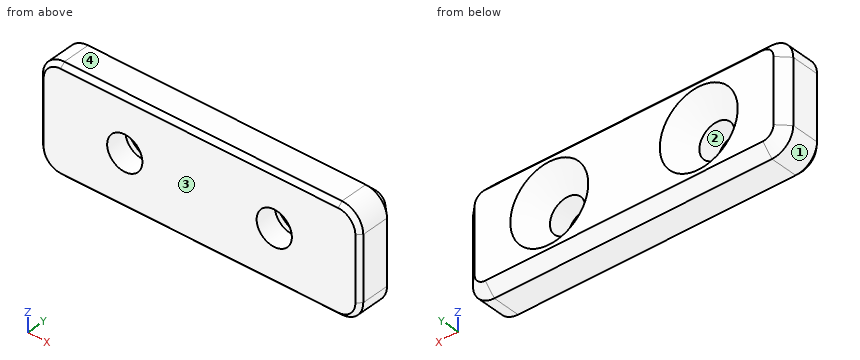
from build123d import *

# Parameters (mm, degrees)
SKETCH_1_W          = 30
SKETCH_1_H          = 10
EXTRUDE_1_DEPTH     = 4
SKETCH_2_R          = 1.65
CUT_EXTRUDE_1_DEPTH = 32.874754901
CHAMFER_1_SIZE      = 2
FILLET_1_R          = 2
CHAMFER_2_SIZE      = 0.4
CHAMFER_3_SIZE      = 1


with BuildPart() as part:
    # 草图1 → 凸台-拉伸1 (new body)
    with BuildSketch(Plane(origin=(0, 0, 0), x_dir=(1, 0, 0), z_dir=(0, 1, 0))):
        with Locations((15, 5)):
            Rectangle(SKETCH_1_W, SKETCH_1_H)
    extrude(amount=EXTRUDE_1_DEPTH)

    # 草图2 → 切除-拉伸1 (cut, through all)
    with BuildSketch(Plane(origin=(0, 4, 0), x_dir=(1, 0, 0), z_dir=(0, 1, 0))):
        with Locations(Location((8, 5, 0), (0, 0, 270))):
            Circle(SKETCH_2_R)
        with Locations(Location((22, 5, 0), (0, 0, 270))):
            Circle(SKETCH_2_R)
    extrude(amount=-CUT_EXTRUDE_1_DEPTH, mode=Mode.SUBTRACT)

    # 倒角1
    chamfer_1_edges = [part.edges().sort_by_distance(p)[0] for p in [
        (8, 4, -6.65),
        (22, 4, -6.65),
    ]]
    chamfer(chamfer_1_edges, length=CHAMFER_1_SIZE)

    # 圆角1
    fillet_1_edges = [part.edges().sort_by_distance(p)[0] for p in [
        (0, 2, -10),
        (30, 2, -10),
        (30, 2, 0),
        (0, 2, 0),
    ]]
    fillet(fillet_1_edges, radius=FILLET_1_R)

    # 倒角2
    chamfer_2_edges = [part.edges().sort_by_distance(p)[0] for p in [
        (15, 0, -10),
        (0, 0, -5),
        (30, 0, -5),
        (15, 0, 0),
        (0.585786438, 0, -9.414213562),
        (0.585786438, 0, -0.585786438),
        (29.414213562, 0, -0.585786438),
        (29.414213562, 0, -9.414213562),
    ]]
    chamfer(chamfer_2_edges, length=CHAMFER_2_SIZE)

    # 倒角3
    chamfer_3_edges = [part.edges().sort_by_distance(p)[0] for p in [
        (15, 4, -10),
        (30, 4, -5),
        (0, 4, -5),
        (15, 4, 0),
        (0.585786438, 4, -9.414213562),
        (0.585786438, 4, -0.585786438),
        (29.414213562, 4, -0.585786438),
        (29.414213562, 4, -9.414213562),
    ]]
    chamfer(chamfer_3_edges, length=CHAMFER_3_SIZE)


solid = part.part
Here's how the part is built. I have some questions about the finished solid (model axes, mm). Face numbers are marked on the shaded views. Round coordinates to 2 decimals unless told otherwise and drop trailing zeros. Order: outer loops, then holes, each group sorted by start corner. A loop starts at its lowest first (then second) coordinate and runs counter-clockwise, first axis right, second up. Notation, with made-up numbers: (39.5, 30) -> (75.5, 30) arc R25 ccw to (75.5, 42) -> close; hole circle Ø8 at (50, 49.25). An arc over 180 degrees is marked (long way). Return JSON: item names as keys, results as strings.
Q1. If we section it at A-A on z = -5: List the corners of the cut face in (x, y) for me, plus the area to 3 significant figures.
Filled sheet:
{"outline": "(0, 0.4) -> (0.4, 0) -> (6.35, 0) -> (6.35, 2) -> (4.35, 4) -> (1, 4) -> (0, 3) -> close; (9.65, 0) -> (20.35, 0) -> (20.35, 2) -> (18.35, 4) -> (11.65, 4) -> (9.65, 2) -> close; (23.65, 0) -> (29.6, 0) -> (30, 0.4) -> (30, 3) -> (29, 4) -> (25.65, 4) -> (23.65, 2) -> close", "area": "84.4 mm^2"}
Q2. If we section it at B-B on x = 8: List the corners of the cut face in (y, z) for me, plus the area to 3 significant figures.
Filled sheet:
{"outline": "(0, -9.6) -> (0.4, -10) -> (3, -10) -> (4, -9) -> (4, -8.65) -> (2, -6.65) -> (0, -6.65) -> close; (0, -3.35) -> (2, -3.35) -> (4, -1.35) -> (4, -1) -> (3, 0) -> (0.4, 0) -> (0, -0.4) -> close", "area": "21.6 mm^2"}
Q3. For pin 1 Ø5.5 at (x, z) = (8, -5) entering from +Y; pin 2 Ø6 at (x, z) = (22.5, -1.5) entering from +Y, each with a flat end and sliding along its axis, tell me the tip position at first contact or that it passes through.
Filled sheet:
{"pin 1": "stops at y = 3.1", "pin 2": "stops at y = 4"}
Q4. If we mould it in two halves opening along Z, with no side actions, what happens to the marked faces 1, 2, 3 and 4? For each: released by +Z, released by -Z, zero draft, split by the parting line, or undercut.
Filled sheet:
{"face 1": "released by -Z", "face 2": "undercut", "face 3": "zero draft", "face 4": "released by +Z"}
Q5. If we section it at D-D on x = 12.5: List the corners of the cut face in (y, z) for me, plus the area to 3 significant figures.
Filled sheet:
{"outline": "(0, -9.6) -> (0.4, -10) -> (3, -10) -> (4, -9) -> (4, -1) -> (3, 0) -> (0.4, 0) -> (0, -0.4) -> close", "area": "38.8 mm^2"}
Q6. I need wall thicknesses on line 1 along X through (y, z) = (1, -5); line 2 along X through (y, z) = (3.4, -3.5); line 3 along Z through (x, y) = (21.5, 3.25). Which ranges of each line are inside material? Lowest first, please. Write a range as from..to.
Filled sheet:
{"line 1": "x = 0..6.35, 9.65..20.35, 23.65..30", "line 2": "x = 0.4..5.34, 10.66..19.34, 24.66..29.6", "line 3": "z = -9.75..-7.86, -2.14..-0.25"}
Q7. If we section it at C-C on y = 0.9: List the corners of the cut face in (x, z) for me.
Filled sheet:
{"outline": "(0, -8) arc R2 ccw to (2, -10) -> (28, -10) arc R2 ccw to (30, -8) -> (30, -2) arc R2 ccw to (28, 0) -> (2, 0) arc R2 ccw to (0, -2) -> close; hole circle Ø3.3 at (8, -5); hole circle Ø3.3 at (22, -5)"}
